```python
from build123d import *

# Parameters (mm, degrees)
SKETCH1_W                  = 80.3
SKETCH1_H                  = 66
BOSS_EXTRUDE1_DEPTH        = 3
FILLET1_R                  = 3.5
F_3_2_3_2_DIAMETER_HOLE1_D = 3.2


with BuildPart() as part:
    # Sketch1 → Boss-Extrude1 (new body)
    with BuildSketch(Plane.XY):
        Polygon((-18, -20), (60.3, -20), (80.3, 0), (0, 0), (0, 66), (-18, 48), align=None)
        with Locations((40.15, 33)):
            Rectangle(SKETCH1_W, SKETCH1_H)
    extrude(amount=BOSS_EXTRUDE1_DEPTH)

    # Fillet1
    fillet1_edges = [part.edges().sort_by_distance(p)[0] for p in [
        (60.3, -20, 1.5),
        (-18, -20, 1.5),
        (-18, 48, 1.5),
        (0, 66, 1.5),
        (80.3, 66, 1.5),
        (80.3, 0, 1.5),
    ]]
    fillet(fillet1_edges, radius=FILLET1_R)

    # Ø3.2 (3.2) Diameter Hole1 (through all)
    with Locations(Plane.XY.offset(3)):
        with Locations((7, 59), (73.3, 59), (73.3, 7), (7, 7)):
            Hole(F_3_2_3_2_DIAMETER_HOLE1_D / 2)


solid = part.part
```
Here's how the part is built. I have some questions about the finished solid (model axes, mm). Coordinates: 2 decimals unless noted, no trailing zeros. Loops run counter-clockwise (first coordinate to the right, second up) from the corner with the lowest first, then second, coordinate; pieces in that order, holes last. Notation, with made-up numbers: (24.25, -13) -> (43.25, -13) arc R25 cw to (43.25, -1) -> close; hole circle Ø8 at (-19, 61.25). An arc over 180 degrees is marked (long way). Return JSON: item names as keys, results as strings.
1) If we section it at C-C, the plane z = 2.4: Write out the boundary of the cut face in (x, y).
Results below:
{"outline": "(-18, -16.5) arc R3.5 ccw to (-14.5, -20) -> (58.85, -20) arc R3.5 ccw to (61.33, -18.97) -> (79.27, -1.03) arc R3.5 ccw to (80.3, 1.45) -> (80.3, 62.5) arc R3.5 ccw to (76.8, 66) -> (1.45, 66) arc R3.5 ccw to (-1.03, 64.97) -> (-16.97, 49.03) arc R3.5 ccw to (-18, 46.55) -> close; hole circle Ø3.2 at (7, 7); hole circle Ø3.2 at (7, 59); hole circle Ø3.2 at (73.3, 7); hole circle Ø3.2 at (73.3, 59)"}
2) I need wall thicknesses on line 1 (Y direction, x = 7, z = 2.3); line 2 (Y direction, x = 73.3, z = 1.75); line 3 (X direction, y = 6, z = 1.3). Which ranges of each line are inside material? Lowest first, please. Write a range as from..to.
Results below:
{"line 1": "-20..5.4, 8.6..57.4, 60.6..66", "line 2": "-7..5.4, 8.6..57.4, 60.6..66", "line 3": "-18..5.75, 8.25..72.05, 74.55..80.3"}
3) Thinking about a two-plate mould opening in X: for faces 1 (the face through (80.3, 32, 1)), 2 (the face through (30, 24, 0)), 3 (the face through (7.35, 5.44, 1.48)), which applies, +X half, -X half, draft (parallel to the pull), parting line (faces both ways), or undercut?
Results below:
{"face 1": "+X half", "face 2": "draft", "face 3": "undercut"}
4) If we section it at A-A, the plane x = 73.3: Write out the boundary of the cut face in (y, z), then the cut area to 3 significant figures.
Results below:
{"outline": "(-7, 0) -> (5.4, 0) -> (5.4, 3) -> (-7, 3) -> close; (8.6, 0) -> (57.4, 0) -> (57.4, 3) -> (8.6, 3) -> close; (60.6, 0) -> (66, 0) -> (66, 3) -> (60.6, 3) -> close", "area": "200 mm²"}
5) If we section it at B-B, the plane y = 7: Write out the boundary of the cut face in (x, z), then the cut area to 3 significant figures.
Results below:
{"outline": "(-18, 0) -> (5.4, 0) -> (5.4, 3) -> (-18, 3) -> close; (8.6, 0) -> (71.7, 0) -> (71.7, 3) -> (8.6, 3) -> close; (74.9, 0) -> (80.3, 0) -> (80.3, 3) -> (74.9, 3) -> close", "area": "276 mm²"}
6) Will this pin go through, and if not, where does the flat tip stop? pin 1 (1.9 mm diameter, centred on x = 73.3, y = 59, fed in from +Z).
Results below:
{"pin 1": "through"}
